```python
from build123d import *

# Parameters (mm, degrees)
F0_R     = 4
F2_R     = 1
F4_T     = -0.5
F5_R     = 2.9
F6_DEPTH = 15


with BuildPart() as f3:
    # F0 (on Top) → F3 section 0
    with BuildSketch(Plane.XY):
        Circle(F0_R)
    # F2 (on offset) → F3 section 1
    with BuildSketch(Plane.XY.offset(18)):
        Circle(F2_R)
    loft()

    # F4
    f4_openings = [f3.faces().sort_by_distance(p)[0] for p in [
        (0, 0, 18),
    ]]
    offset(amount=F4_T, openings=f4_openings, kind=Kind.INTERSECTION)

    # F5 (on face) → F6 (join)
    with BuildSketch(Plane(origin=(0, 0, 0), x_dir=(1, 0, 0), z_dir=(0, 0, -1))):
        Circle(F5_R)
    extrude(amount=F6_DEPTH)


solid = f3.part
```
Could you check a few things on this model? Use its own coordinates, in mm. A direction names the side the tool comes from. Round coordinates to 2 decimals unless told otherwise and drop trailing zeros. Order: outer loops, then holes, each group sorted by start corner. A loop starts at its lowest first (then second) coordinate and runs counter-clockwise, first axis right, second up. Notation, with made-up numbers: (-11, -1.5) -> (-7, -1.5) arc R26 ccw to (-7, 15.5) -> close; hole circle Ø3 at (15, 48.25). An arc over 180 degrees is marked (long way). One line per question, with ' | ' between items.
Q1. I'm going to push flat-ended pins straight in: pin 1 (2 mm diameter, centred on x = 2.5, z = 1, fed in from +Y); pin 2 (1 mm diameter, centred on x = 2.5, z = -9, fed in from +Y); pin 3 (1 mm diameter, centred on x = -2.5, z = 9.5, fed in from -Y). Where does each tip first touch, or does it pass through?
Computed values:
pin 1: y = 3.56 | pin 2: y = 2.1 | pin 3: y = -1.37
Q2. If we section it at B-B on z = -6: Write out the boundary of the cut face in (x, y), plus the area to 3 significant figures.
Computed values:
outline: circle Ø5.8 at (0, 0) | area: 26.4 mm²
Q3. We'd pull the mould along X, two halves only. Please class faces 3 (the face through (-0.54, -2.42, 9.13)), 4 (the face through (0, 0, -15)), 5 (the face through (0, 0, 0.5)): released by +X, released by -X, zero draft, split by the parting line, or undercut.
Computed values:
face 3: split by the parting line | face 4: zero draft | face 5: undercut
Q4. If we section it at C-C on z = 3: Write out the boundary of the cut face in (x, y), plus the area to 3 significant figures.
Computed values:
outline: circle Ø7 at (0, 0); hole circle Ø5.99 at (0, 0) | area: 10.3 mm²
Q5. If we section it at A-A on x = 0: Write out the boundary of the cut face in (y, z), plus the area to 3 significant figures.
Computed values:
outline: (-4, 0) -> (-2.9, 0) -> (-2.9, -15) -> (2.9, -15) -> (2.9, 0) -> (4, 0) -> (1, 18) -> (0.49, 18) -> (3.41, 0.5) -> (-3.41, 0.5) -> (-0.49, 18) -> (-1, 18) -> close | area: 109 mm²
Q6. If I drill on line 1 (X direction, y = 0.25, z = 15); line 2 (X direction, y = 1.25, z = 7.5); line 3 (Y direction, x = 0.5, z = 13), over which ranges is the centre line in solid material (lowest first)? Write a range as from..to.
Computed values:
line 1: -1.48..-0.96, 0.96..1.48 | line 2: -2.45..-1.86, 1.86..2.45 | line 3: -1.76..-1.23, 1.23..1.76
Q7. If we section it at D-D on z = 9.5: Write out the boundary of the cut face in (x, y).
Computed values:
outline: circle Ø4.83 at (0, 0); hole circle Ø3.82 at (0, 0)
Q8. Which directions (+Z, -Z, +X, -X, +Y, -Y) give clear straight access to the entire face, cutting with the end or side of a thin tool? Please do faces 1 (the face through (-1.532, -1.175, 9.372)), 2 (the face through (-2.9, -0.1, -7.4)).
Computed values:
face 1: none | face 2: -Z
